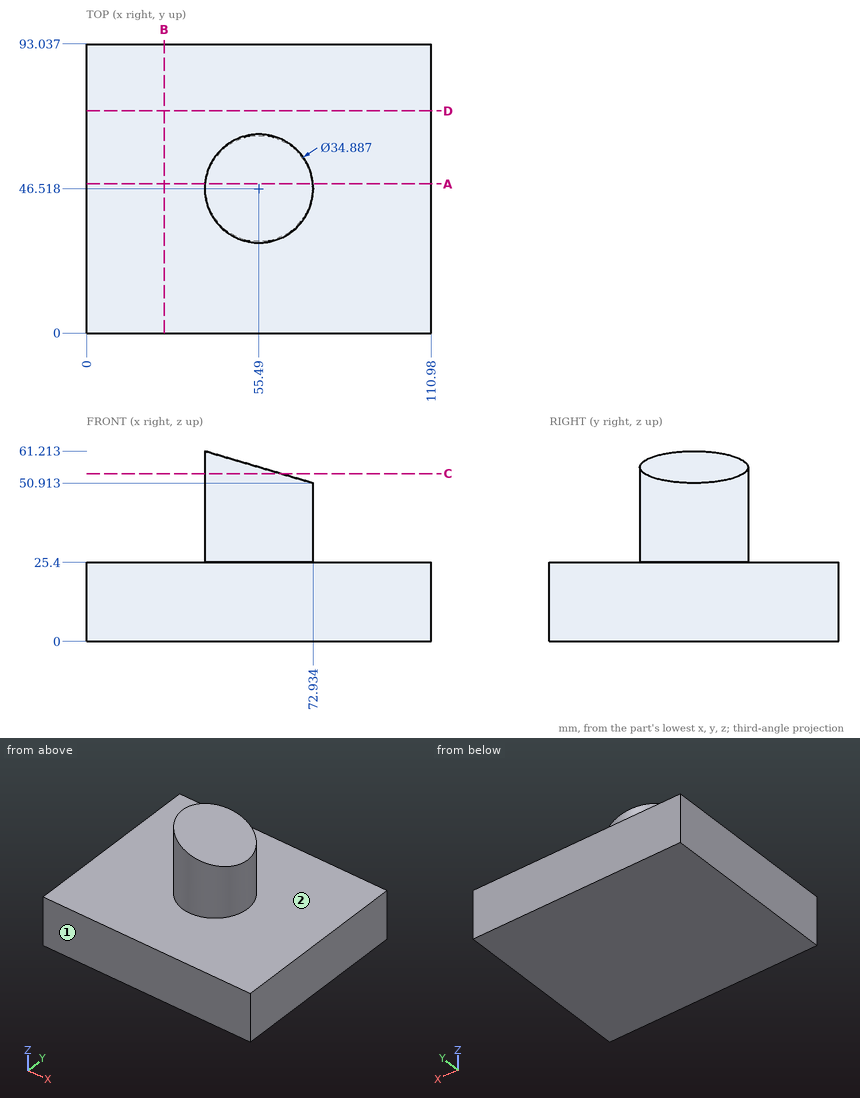
Job drawing, mm, ordinate dimensions from the low corner. One solid piece. A direction names the side the tool comes from. Coordinates: 2 decimals unless noted, no trailing zeros. Loops run counter-clockwise (first coordinate to the right, second up) from the corner with the lowest first, then second, coordinate; pieces in that order, holes last. Notation, with made-up numbers: (25.25, 15.5) - (48.25, 15.5) arc R28 cw to (48.25, 43.5) - close; hole circle Ø8 at (-28, 67.5). An arc over 180 degrees is marked (long way). Write item = value, one per line. Start each with the question number.
Q1. Flat gauge pins, fed straight in: pin 1 Ø1.5 at (y, z) = (45, 28) entering from -X; pin 2 Ø10 at (y, z) = (42.5, 32.5) entering from -X. Where does each tip first touch, or does it go through?
Q2. Cut at B-B, the plane x = 25. List the corners of the cut face in (y, z).
Q3. Cut at D-D, the plane y = 71.5. List the corners of the cut face in (x, z), then the cut area to 3 significant figures.
Q4. Cut at C-C, the plane z = 54. List the corners of the cut face in (x, y) (1 decimal).
Q5. Cut at A-A, the plane y = 48. List the corners of the cut face in (x, z) (1 decimal).
Q6. Drill centre lines: L1, parallel to Z at x = 15, y = 27.5; L2, parallel to X at y = 46, z = 27 (1 decimal); L3, parallel to X at y = 39.5, z = 48. Where is each one in solid material? Low to high.
Q7. Which spindle directions (+Z, -Z, +X, -X, +Y, -Y) get a long thin tool onto all of the face, cutting with end or side? Do the marked faces 1 and 2. Say none if no direction does.
Computed:
q1.pin_1 = 38.06
q1.pin_2 = 38.05
q2.outline = (0, 0) - (93.04, 0) - (93.04, 25.4) - (0, 25.4) - close
q3.outline = (0, 0) - (110.98, 0) - (110.98, 25.4) - (0, 25.4) - close
q3.area = 2,820 mm²
q4.outline = (62.5, 30.5) - (62.5, 62.5) arc R17.4 ccw (long way) to start
q5.outline = (0, 0) - (111, 0) - (111, 25.4) - (72.9, 25.4) - (72.9, 50.9) - (38.1, 61.2) - (38.1, 25.4) - (0, 25.4) - close
q6.L1 = 0 to 25.4
q6.L2 = 38.1 to 72.9
q6.L3 = 39.52 to 71.46
q7.face_1 = +Z, -Z, +X, -X, -Y
q7.face_2 = +Z
